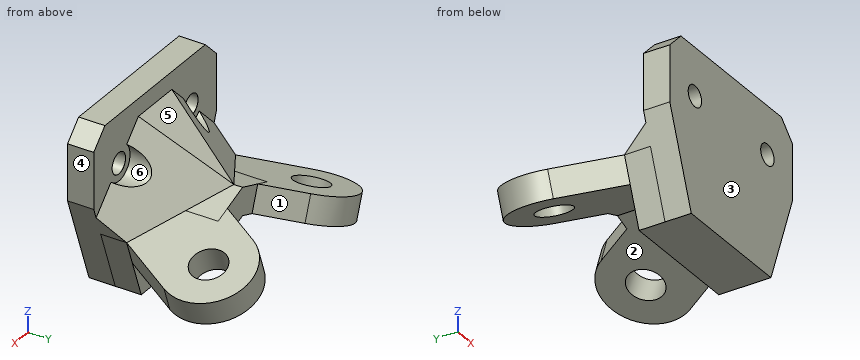
```python
from build123d import *

# Parameters (mm, degrees)
SKETCH1_W                           = 110
SKETCH1_H                           = 95
BOSS_EXTRUDE1_DEPTH                 = 15
SKETCH6_R                           = 25
SKETCH6_R_2                         = 10
BOSS_EXTRUDE7_DEPTH                 = 15
DELETEFACE4_START                   = 15
DELETEFACE4_DEPTH                   = 50
CUT_EXTRUDE1_DEPTH                  = 29.85315
BOSS_EXTRUDE8_DEPTH                 = 14.85315
F_12_0_12_DIAMETER_HOLE1_AT_2_COUNT = 2
F_12_0_12_DIAMETER_HOLE1_AT_2_PITCH = 65
SKETCH17_R                          = 10
CUT_EXTRUDE2_DEPTH                  = 15
CHAMFER1_SIZE                       = 10


# Read off the part's stored shape, not the designer's step: DeleteFace4
with BuildPart() as part:
    # Sketch1 → Boss-Extrude1 (new body)
    with BuildSketch(Plane(origin=(0, 0, 0), x_dir=(1, 0, 0), z_dir=(0, 1, 0))):
        with Locations((0, 47.5)):
            Rectangle(SKETCH1_W, SKETCH1_H)
    extrude(amount=BOSS_EXTRUDE1_DEPTH)

    # Sketch6 → Boss-Extrude7 (add)
    # profile 1 of 3: a face of its own
    with BuildSketch(Plane(origin=(-46.172719349, 75, -58.141496194), x_dir=(0.9396926207859081, 0, 0.34202014332566977), z_dir=(-0.3420201433256697, 0, 0.939692620785908))):
        Circle(SKETCH6_R)
        Circle(SKETCH6_R_2, mode=Mode.SUBTRACT)
    # profile 2 of 3: a face of its own
    with BuildSketch(Plane(origin=(-46.172719349, 75, -58.141496194), x_dir=(0.9396926207859081, 0, 0.34202014332566977), z_dir=(-0.3420201433256697, 0, 0.939692620785908))):
        with BuildLine():
            ThreePointArc((25, 0), (6.470476128, -24.148145657), (-21.650635095, -12.5))
            Line((-21.650635095, -12.5), (5.773502692, -60))
            Line((5.773502692, -60), (63.508529611, -60))
            Line((63.508529611, -60), (34.641016151, -10))
            Line((34.641016151, -10), (21.650635095, 12.5))
            ThreePointArc((21.650635095, 12.5), (24.148145657, 6.470476128), (25, 0))
        make_face()
    # profile 3 of 3: a face of its own
    with BuildSketch(Plane(origin=(-46.172719349, 75, -58.141496194), x_dir=(0.9396926207859081, 0, 0.34202014332566977), z_dir=(-0.3420201433256697, 0, 0.939692620785908))):
        Polygon((34.641016151, -10), (63.508529611, -60), (84.985310553, -60), (84.985310553, -10), align=None)
    boss_extrude7 = extrude(amount=-BOSS_EXTRUDE7_DEPTH)

    # Mirror1: Boss-Extrude7 across plane
    add(boss_extrude7.mirror(Plane(origin=(0, 0, 0), x_dir=(0, 0, 1), z_dir=(1, 0, 0))))

    # DeleteFace4 outline → DeleteFace4 (cut)
    with BuildSketch(Plane(origin=(0, 0, 0), x_dir=(1, 0, 0), z_dir=(0, 1, 0)).offset(DELETEFACE4_START)):
        Polygon((21.928533001, 49.317334009), (0, 41.336000716), (33.687349853, 29.074808098), (38.817652003, 43.17019741), align=None)
        Polygon((0, 41.336000716), (-21.928533001, 49.317334009), (-38.817652003, 43.17019741), (-33.687349853, 29.074808098), align=None)
    extrude(amount=DELETEFACE4_DEPTH, mode=Mode.SUBTRACT)

    # Sketch8 → Loft1 section 0
    with BuildSketch(Plane(origin=(0, 15, 0), x_dir=(1, 0, 0), z_dir=(0, 1, 0)), mode=Mode.PRIVATE) as loft1_s0:
        with BuildLine():
            Line((-15, 10), (15, 10))
            Line((15, 10), (72.85193746, 67.85193746))
            Line((72.85193746, 67.85193746), (0, 41.336000716))
            Line((0, 41.336000716), (-72.85193746, 67.85193746))
            Line((-72.85193746, 67.85193746), (-15, 10))
        make_face()
    loft([Vertex(0, 60, -41.336000716), loft1_s0.sketch])

    # Sketch13 → Cut-Extrude1 (cut)
    with BuildSketch(Plane(origin=(0, 0, 0), x_dir=(1, 0, 0), z_dir=(0, 1, 0))):
        Polygon((-55, 95), (-55, 42.081139662), (-35.739110006, 95), align=None)
    extrude(amount=CUT_EXTRUDE1_DEPTH, mode=Mode.SUBTRACT)


with BuildPart() as cut_extrude1_kept_piece:
    # of the separate pieces the step leaves, the one the design keeps (cut_extrude1_pieces_kept)
    add(part.part.solids().sort_by_distance((-55, 0, 0))[0])

    # Sketch14 → Boss-Extrude8 (add)
    with BuildSketch(Plane(origin=(0, 15, 0), x_dir=(1, 0, 0), z_dir=(0, 1, 0))):
        Polygon((0, 57.298667303), (0, 95), (-35.739110006, 95), (-48.805705227, 59.099824681), (-40.747401473, 56.166841976), (-35.617099323, 70.262231288), align=None)
    extrude(amount=BOSS_EXTRUDE8_DEPTH)

    # SurfaceCut2
    split(bisect_by=Plane(origin=(0, 0, 0), x_dir=(0, 0, -1), z_dir=(1, 0, 0)), keep=Keep.BOTTOM)

    # Mirror3: Cut-Extrude1 kept piece across plane


with BuildPart() as cut_extrude1_kept_piece_1:
    add(cut_extrude1_kept_piece.part)
    add(cut_extrude1_kept_piece.part.mirror(Plane(origin=(0, 0, 0), x_dir=(0, 0, 1), z_dir=(1, 0, 0))))

    # Sketch16 → Ø12.0 (12) Diameter Hole1 (revolve, cut)
    with BuildSketch(Plane(origin=(32.5, 15, -27.5), x_dir=(0, 0, 1), z_dir=(1, 0, 0))):
        Polygon((0, 0), (0, 15), (6, 15), (6, 0.025), (6.025, 0), align=None)
    f_12_0_12_diameter_hole1 = revolve(axis=Axis((32.5, 21.35, -27.5), (0, -1, 0)), mode=Mode.SUBTRACT)

    # Ø12.0 (12) Diameter Hole1 at 2: Ø12.0 (12) Diameter Hole1 ×2
    with Locations(*[(-i * F_12_0_12_DIAMETER_HOLE1_AT_2_PITCH, 0, 0) for i in range(1, F_12_0_12_DIAMETER_HOLE1_AT_2_COUNT)]):
        add(f_12_0_12_diameter_hole1, mode=Mode.SUBTRACT)

    # Sketch17 → Cut-Extrude2 (cut)
    with BuildSketch(Plane(origin=(0, 15, 0), x_dir=(1, 0, 0), z_dir=(0, 1, 0))):
        with Locations((-32.5, 27.5)):
            Circle(SKETCH17_R)
        with Locations((32.5, 27.5)):
            Circle(SKETCH17_R)
    extrude(amount=CUT_EXTRUDE2_DEPTH, mode=Mode.SUBTRACT)

    # Chamfer1
    chamfer1_edges = [cut_extrude1_kept_piece_1.edges().sort_by_distance(p)[0] for p in [
        (-55, 7.5, 0),
        (55, 7.5, 0),
    ]]
    chamfer(chamfer1_edges, length=CHAMFER1_SIZE)


solid = cut_extrude1_kept_piece_1.part
```
Can you work these out from the model? Positions are in its coordinate system, mm. Face numbers are marked on the shaded views. A direction names the side the tool comes from. Coordinates: 2 decimals unless noted, no trailing zeros. Write each loop counter-clockwise with the first axis right and the second up, starting at its lowest first coordinate (ties: lowest second). Pieces come first, ordered by that corner, then holes. Notation, with made-up numbers: M -2.5,76.5 L 21.5,76.5 A9 ccw 21.5,93.5 Z; hole C 34,32 d9. An arc over 180 degrees is marked long. Write item = value, one per line. Start each with the question number.
Q1. If we section it at A-A, the plane y = 70.5: Write out the boundary of the cut face in (x, z).
Q2. I'm going to push flat-ended pins straight in: pin 1 (15 mm diameter, centred on x = -1.5, z = -51, fed in from +Y); pin 2 (6 mm diameter, centred on y = 18.5, z = -68, fed in from -X); pin 3 (19 mm diameter, centred on x = -32.5, z = -27.5, fed in from +Y). Where does each tip first touch, or does it pass through?
Q3. If we section it at C-C, the plane y = 8: Write out the boundary of the cut face in (x, z).
Q4. If we section it at D-D, the plane x = -4: Write out the boundary of the cut face in (y, z), then the cut area to 3 significant figures.
Q5. Thinking about a two-plate mould opening in X: for the marked faces 4, 5 and 6, which applies, released by +X, released by -X, zero draft, split by the parting line, or undercut?
Q6. On a 3-axis mill with a long thin cutter (end or side, diameter ignored), from which of +Z, -Z, +X, -X, +Y, -Y can I reach the whole of each face in a straight line? I mean the marked faces 1, 2 and 3. Say none if no direction works.
Q7. If I drill on L1, parallel to X at y = 11, z = -27.5; L2, parallel to Z at x = 32.5, y = 8.5; L3, parallel to Y at x = 39, z = -6.5, over which ranges is the centre line in solid material (lowest first)? Write a range as [from, to].
Q8. If we section it at B-B, the plane z = -27.5: Write out the boundary of the cut face in (x, y) (3 decimals), then the cut area to 3 significant figures.
Check sheet entries:
q1.outline = M -69.28,-66.55 L -64.15,-80.65 L -49.43,-75.29 L -54.56,-61.2 Z; M -37.78,-55.09 L -32.65,-69.18 L -11.47,-61.48 L -16.6,-47.38 Z; M 11.47,-61.48 L 32.65,-69.18 L 37.78,-55.09 L 16.6,-47.38 Z; M 49.43,-75.29 L 64.15,-80.65 L 69.28,-66.55 L 54.56,-61.2 Z
q2.pin_1 = 65
q2.pin_2 = -46.66
q2.pin_3 = 15
q3.outline = M -55,-42.08 L -35.74,-95 L 35.74,-95 L 55,-42.08 L 55,-10 L 45,0 L -45,0 L -55,-10 Z; hole C -32.5,-27.5 d12; hole C 32.5,-27.5 d12
q4.outline = M 0,-95 L 29.85,-95 L 29.85,-58.75 L 65,-58.75 L 65,-42.79 L 57.53,-42.79 L 48,-32.98 L 15,-10 L 15,0 L 0,0 Z
q4.area = 3,510 mm²
q5.face_4 = released by +X
q5.face_5 = zero draft
q5.face_6 = undercut
q6.face_1 = +Z, +Y
q6.face_2 = -Z, +Y
q6.face_3 = +Z, -Z, +X, -X, -Y
q7.L1 = [-55, -38.5], [-26.5, 26.5], [38.5, 55]
q7.L2 = [-95, -33.5], [-21.5, 0]
q7.L3 = [0, 15]
q8.outline = M -55,0 L -38.5,0 L -38.5,14.975 L -38.525,15 L -55,15 Z; M -26.5,0 L 26.5,0 L 26.5,14.975 L 26.475,15 L 22.5,15 L 22.5,24.712 L 6.623,40.131 L -6.623,40.131 L -22.5,24.712 L -22.5,15 L -26.475,15 L -26.5,14.975 Z; M 38.5,0 L 55,0 L 55,15 L 38.525,15 L 38.5,14.975 Z
q8.area = 2,180 mm²
